The drawing under review shows one solid part. Ordinate dimensions are in mm from its lowest x, y, z. A direction names the side the tool comes from. Coordinates: 2 decimals unless noted, no trailing zeros. Write each loop counter-clockwise with the first axis right and the second up, starting at its lowest first coordinate (ties: lowest second). Pieces come first, ordered by that corner, then holes.
Q1. The part is to be moulded in two halves that separate along Z. For the marked faces 1, 2, 3 and 4, say which applies: +Z half, -Z half, draft (parallel to the pull), parting line (faces both ways), or undercut.
Q2. Clearance check with flat-ended pins moving along their axes: pin 1 Ø1 at (x, y) = (29.5, 3) entering from +Z; pin 2 Ø2 at (x, y) = (13.5, 5.5) entering from -Z (1 decimal); pin 3 Ø3 at (x, y) = (37.5, 4) entering from -Z (1 decimal); pin 4 Ø2 at (x, z) = (30.12, 30.12) entering from +Y. State where each tip first meets the part, or that it passes through.
Q3. Add section B-B, the plane y = 6.25. Give the number of separate pieces and of enclosed holes in the cut face, plus the area to 3 significant figures.
Q4. Machinability: for the marked faces 5, 6 and 7, which of the approach directions +Z, -Z, +X, -X, +Y, -Y give a long, thin tool a straight path to every point of the face, cutting with its end or side? Answer none if there is none.
Q5. To check wall thickness, follow probe 1 along X at (y, z) = (3, 11) (1 decimal); probe 2 along X at (y, z) = (1, 2.5); probe 3 along Z at (x, y) = (3, 4.5) (1 decimal). State the ranges of each line that lie inside material, in increasing order.
Q6. Add section A-A, the plane z = 20. Give the boundary of the cut face in (x, y) (1 decimal), plus the area to 3 significant figures.
Q7. Add section C-C, the plane x = 7.5. Give the boundary of the cut face in (y, z).
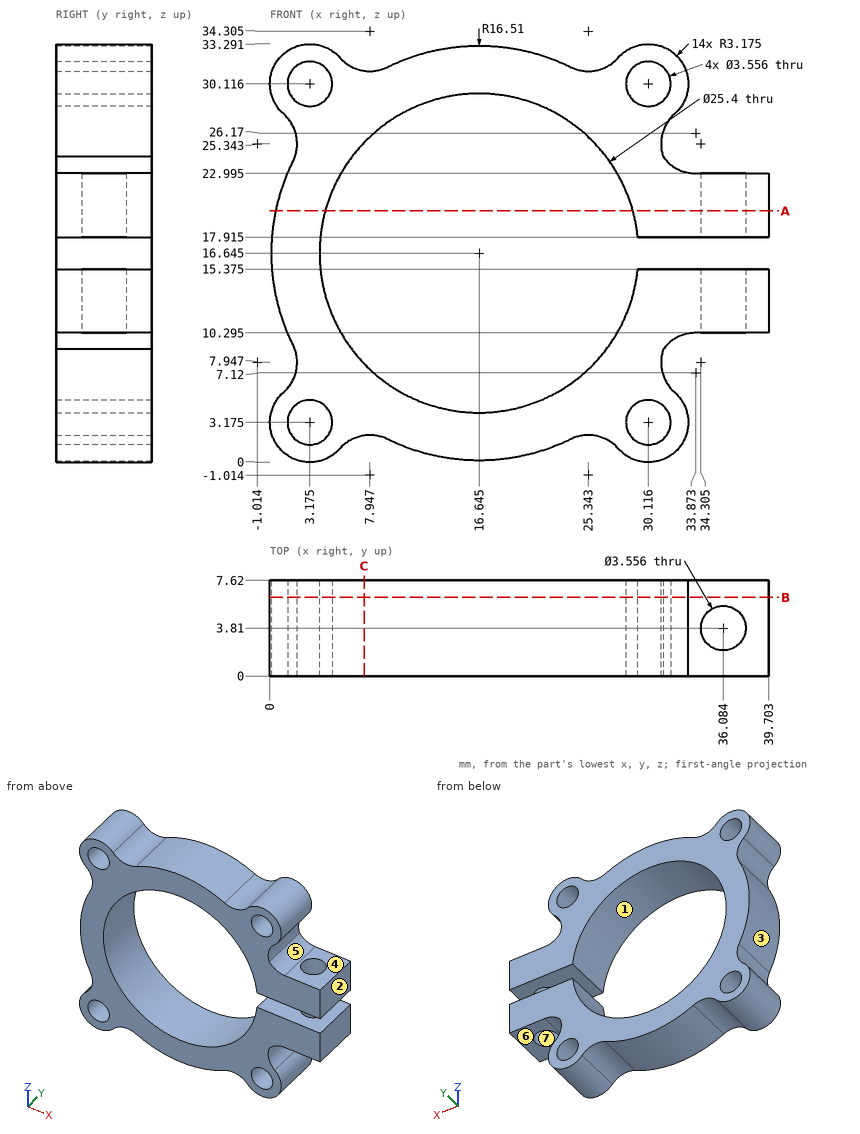
Here are the results:
1. face 1: undercut
1. face 2: draft
1. face 3: undercut
1. face 4: +Z half
2. pin 1: stops at z = 33.29
2. pin 2: stops at z = 0.3
2. pin 3: stops at z = 10.3
2. pin 4: passes through
3. separate pieces: 1
3. enclosed holes: 4
3. area: 512 mm2
4. face 5: +X, +Y, -Y
4. face 6: -Z, +X, +Y, -Y
4. face 7: +Z, -Z
5. probe 1: x = 1.1 to 5.3, 28 to 34.5, 37.7 to 39.7
5. probe 2: x = 0.07 to 1.53, 4.82 to 28.47, 31.76 to 33.22
5. probe 3: z = 0 to 1.4, 4.9 to 28.3, 31.9 to 33.3
6. outline: (0.5, 0) - (4.4, 0) - (4.4, 7.6) - (0.5, 7.6) - close; (28.9, 0) - (39.7, 0) - (39.7, 7.6) - (28.9, 7.6) - close; hole circle Ø3.6 at (36.1, 3.8)
6. area: 102 mm2
7. outline: (0, 2.13) - (7.62, 2.13) - (7.62, 7.83) - (0, 7.83) - close; (0, 25.46) - (7.62, 25.46) - (7.62, 31.16) - (0, 31.16) - close
